```python
from build123d import *

# Parameters (mm, degrees)
TROU_TARAUD_M2_51_D     = 2.05
TROU_TARAUD_M2_51_DEPTH = 9.25
TROU_TARAUD_M2_51_TIP   = 0.615882135
CONG_1_R                = 0.2


with BuildPart() as part:
    # Esquisse1 → Révolution1 (revolve)
    with BuildSketch(Plane.XY, mode=Mode.PRIVATE) as r_volution1_sk:
        Polygon((0, 25.6), (4, 25.6), (4, 20), (3, 20), (3, 0), (0, 0), align=None)
    revolve(r_volution1_sk.sketch.rotate(Axis((0, 0, 0), (0, 1, 0)), 90), axis=Axis((0, 0, 0), (0, 1, 0)))

    # Trou taraudé M2.51
    with Locations(Plane(origin=(0, 0, 0), x_dir=(-1, 0, 0), z_dir=(0, -1, 0))):
        with Locations((0, 0)):
            Hole(TROU_TARAUD_M2_51_D / 2, depth=TROU_TARAUD_M2_51_DEPTH)
            with Locations((0, 0, -(TROU_TARAUD_M2_51_DEPTH + TROU_TARAUD_M2_51_TIP / 2))):  # 118° drill point
                Cone(0, TROU_TARAUD_M2_51_D / 2, TROU_TARAUD_M2_51_TIP, mode=Mode.SUBTRACT)

    # Congé1
    cong_1_edges = [part.edges().sort_by_distance(p)[0] for p in [
        (0, 0, 3),
        (0, 20, 4),
        (0, 25.6, 4),
    ]]
    fillet(cong_1_edges, radius=CONG_1_R)


solid = part.part
```
Verification items for the finished model (mm, model axes). A direction names the side the tool comes from. Give positions to 0.01 mm unless a question says otherwise; leave off trailing zeros. Order: outer loops, then holes, each group sorted by start corner. A loop starts at its lowest first (then second) coordinate and runs counter-clockwise, first axis right, second up. Notation, with made-up numbers: M 20.5,57.25 L 44.5,57.25 A16 cw 44.5,79.25 Z; hole C -28.75,13 d7. An arc over 180 degrees is marked long. Return JSON: item names as keys, results as strings. Group by question number.
1) Mould release check, pull along X, two halves, no side actions. Record for faces 1 (the face through (-0.133, 4.69, -1.016)), 2 (the face through (-0.9, 9.96, -2.86)), 3 (the face through (0, 25.6, 0)): pulls with the +X half, pulls with the -X half, needs draft (parallel to the pull), parting line crosses it, or undercut.
2) Section check B-B on y = 21.5. Record the cut outline in (x, z), and give its area (3 significant figures).
3) Go/stop test with flat-tipped pins: pin 1 Ø3 at (y, z) = (3.5, 3) entering from -X; pin 2 Ø1 at (y, z) = (21, 1) entering from +X. Record where each tip stops, or that it passes through.
4) Section check A-A on y = 13. Record the cut outline in (x, z), and give its area (3 significant figures).
5) Scan lines: line 1 (Y direction, x = -2.75, z = -2.25); line 2 (X direction, y = 1, z = 0.75); line 3 (Z direction, x = 1.25, y = 10.5). Record each from-to range of solid material in increasing order.
6) Access from +Z, -Z, +X, -X, +Y, -Y to the whole of each face (thin tool, end or side, straight path). Record for faces 4 (the face through (-1, 20, -3)), 5 (the face through (0, 0, -1.2)).
Answer block:
{
 "1": {"face 1": "undercut", "face 2": "parting line crosses it", "face 3": "needs draft"},
 "2": {"outline": "C 0,0 d8", "area": "50.3 mm^2"},
 "3": {"pin 1": "stops at x = -2.6", "pin 2": "stops at x = 3.97"},
 "4": {"outline": "C 0,0 d6", "area": "28.3 mm^2"},
 "5": {"line 1": "y = 20 to 25.6", "line 2": "x = -2.9 to -0.7, 0.7 to 2.9", "line 3": "z = -2.73 to 2.73"},
 "6": {"face 4": "-Y", "face 5": "+Z, -Z, +X, -X, -Y"}
}
